```python
from build123d import *

# Parameters (mm, degrees)
SKETCH_R        = 5
SKETCH_R_2      = 3.2
PAD_DEPTH       = 15
SKETCH002_R     = 6.1
POCKET001_DEPTH = 4
SKETCH003_R     = 11.1
POCKET_DEPTH    = 7.4


with BuildPart() as part:
    # Sketch → Pad (new body)
    with BuildSketch(Plane.XY):
        Polygon((20, 30), (20, 51), (62.3, 51), (62.3, 30), (82.3, 30), (82.3, 0), (0, 0), (0, 30), align=None)
        with Locations((41.15, 29.85)):
            Circle(SKETCH_R, mode=Mode.SUBTRACT)
        with Locations((11.15, 10)):
            Circle(SKETCH_R_2, mode=Mode.SUBTRACT)
        with Locations((31.15, 10)):
            Circle(SKETCH_R_2, mode=Mode.SUBTRACT)
        with Locations((51.15, 10)):
            Circle(SKETCH_R_2, mode=Mode.SUBTRACT)
        with Locations((71.15, 10)):
            Circle(SKETCH_R_2, mode=Mode.SUBTRACT)
    extrude(amount=PAD_DEPTH)

    # Sketch002 → Pocket001 (cut)
    with BuildSketch(Plane(origin=(0, 0, 0), x_dir=(1, 0, 0), z_dir=(0, 0, -1))):
        with Locations((11.15, -10)):
            Circle(SKETCH002_R)
        with Locations((31.15, -10)):
            Circle(SKETCH002_R)
        with Locations((51.15, -10)):
            Circle(SKETCH002_R)
        with Locations((71.15, -10)):
            Circle(SKETCH002_R)
    extrude(amount=-POCKET001_DEPTH, mode=Mode.SUBTRACT)

    # Sketch003 (on Face5 of Pocket001) → Pocket (cut)
    with BuildSketch(Plane.XY.offset(15)):
        with Locations((41.15, 29.85)):
            Circle(SKETCH003_R)
    extrude(amount=-POCKET_DEPTH, mode=Mode.SUBTRACT)


solid = part.part
```
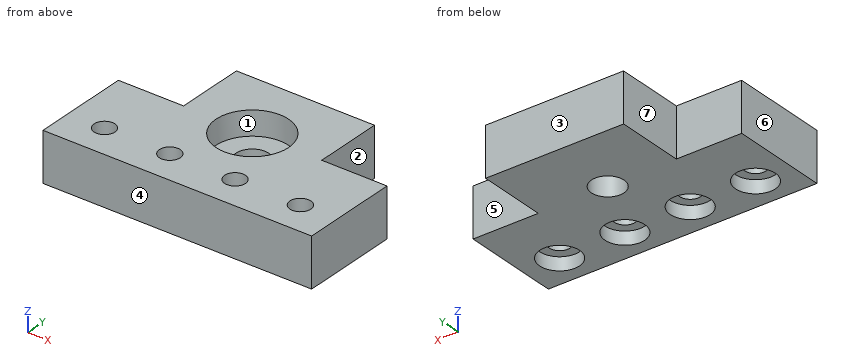
For this review, take the finished solid that the model builds, in its own axes (mm). Face numbers are marked on the shaded views. A direction names the side the tool comes from. Coordinates: 2 decimals unless noted, no trailing zeros. Write each loop counter-clockwise with the first axis right and the second up, starting at its lowest first coordinate (ties: lowest second). Pieces come first, ordered by that corner, then holes.
(1) Tool access review of the marked faces 5, 6 and 7: name each direction out of +Z, -Z, +X, -X, +Y, -Y from which nothing blocks a thin tool from reaching the whole face with its end or side.
(2) For pin 1 Ø10 at (x, y) = (21.5, 17.5) entering from -Z; pin 2 Ø1 at (x, y) = (54.5, 9.5) entering from -Z; pin 3 Ø7.5 at (y, z) = (37, 7) entering from -X; pin 4 Ø7.5 at (x, z) = (74.5, 5.5) entering from +Y, all flat-tipped, find the tip position at first contact; note any pin that passes through.
(3) Add section C-C on y = 31.5. Give the boundary of the cut face in (x, z), then the cut area to 3 significant figures.
(4) Add section B-B on x = 71.15. Give the boundary of the cut face in (y, z).
(5) Add section D-D on z = 13.25. Give the boundary of the cut face in (x, y), then the cut area to 3 significant figures.
(6) Add section A-A on z = 5. Give the boundary of the cut face in (x, y), then the cut area to 3 significant figures.
(7) The part is to be moulded in two halves that separate along Y. For the marked faces 1, 2, 3 and 4, say which applies: +Y half, -Y half, draft (parallel to the pull), parting line (faces both ways), or undercut.
(8) Wall thickness on probe 1 along X at (y, z) = (10, 11.75); probe 2 along X at (y, z) = (10, 1.35); probe 3 along Y at (x, z) = (31.15, 9.25): over which ranges is each line inside the solid? List them lowest first.
Answer sheet:
1. face 5: +Z, -Z, +X, +Y
1. face 6: +Z, -Z, -X, +Y, -Y
1. face 7: +Z, -Z, -X, +Y
2. pin 1: stops at z = 0
2. pin 2: stops at z = 4
2. pin 3: stops at x = 20
2. pin 4: stops at y = 30
3. outline: (20, 0) - (36.43, 0) - (36.43, 7.6) - (30.17, 7.6) - (30.17, 15) - (20, 15) - close; (45.87, 0) - (62.3, 0) - (62.3, 15) - (52.13, 15) - (52.13, 7.6) - (45.87, 7.6) - close
3. area: 400 mm2
4. outline: (0, 0) - (3.9, 0) - (3.9, 4) - (6.8, 4) - (6.8, 15) - (0, 15) - close; (13.2, 4) - (16.1, 4) - (16.1, 0) - (30, 0) - (30, 15) - (13.2, 15) - close
5. outline: (0, 0) - (82.3, 0) - (82.3, 30) - (62.3, 30) - (62.3, 51) - (20, 51) - (20, 30) - (0, 30) - close; hole circle Ø6.4 at (11.15, 10); hole circle Ø6.4 at (31.15, 10); hole circle Ø22.2 at (41.15, 29.85); hole circle Ø6.4 at (51.15, 10); hole circle Ø6.4 at (71.15, 10)
5. area: 2,840 mm2
6. outline: (0, 0) - (82.3, 0) - (82.3, 30) - (62.3, 30) - (62.3, 51) - (20, 51) - (20, 30) - (0, 30) - close; hole circle Ø6.4 at (11.15, 10); hole circle Ø6.4 at (31.15, 10); hole circle Ø10 at (41.15, 29.85); hole circle Ø6.4 at (51.15, 10); hole circle Ø6.4 at (71.15, 10)
6. area: 3,150 mm2
7. face 1: undercut
7. face 2: draft
7. face 3: +Y half
7. face 4: -Y half
8. probe 1: x = 0 to 7.95, 14.35 to 27.95, 34.35 to 47.95, 54.35 to 67.95, 74.35 to 82.3
8. probe 2: x = 0 to 5.05, 17.25 to 25.05, 37.25 to 45.05, 57.25 to 65.05, 77.25 to 82.3
8. probe 3: y = 0 to 6.8, 13.2 to 25.03, 34.67 to 51
